Could you check a few things on this model? Use its own coordinates, in mm. Round coordinates to 2 decimals unless told otherwise and drop trailing zeros. Loops run counter-clockwise (first coordinate to the right, second up) from the corner with the lowest first, then second, coordinate; pieces in that order, holes last. Notation, with made-up numbers: M 45.25,41.25 L 50.25,41.25 A14 cw 50.25,54.25 Z; hole C -22.75,20 d8. An arc over 180 degrees is marked long. One line per item, written item: value. Start each with the question number.
Q1. Please list where these lines run through material, in increasing order: line 1 along X through (y, z) = (1.6, -32); line 2 along X through (y, z) = (1.35, -20.37); line 3 along X through (y, z) = (3, 19.63).
Q2. Imagine slicing it at D-D (z = 32). Please give me the cut outline in (x, y).
Q3. I'm going to push flat-ended pins straight in: pin 1 Ø2.5 at (x, z) = (58.87, -20.37) entering from +Y; pin 2 Ø2.5 at (x, y) = (-37.5, 1.5) entering from +Z; pin 3 Ø2.5 at (x, y) = (54.5, 3.5) entering from -Z; pin 4 Ø2.5 at (x, y) = (-70.5, 1.5) entering from -Z. Where does each tip first touch, or does it pass through?
Q4. Imagine slicing it at A-A (x = 1.5). Please give me the cut outline in (y, z), then the cut area to 3 significant figures.
Q5. Imagine slicing it at B-B (y = 3.3). Give the number of separate pieces and of enclosed holes in the cut face, then the cut area to 3 significant figures.
Q6. Imagine slicing it at C-C (x = 58.87). Please give me the cut outline in (y, z), then the cut area to 3 significant figures.
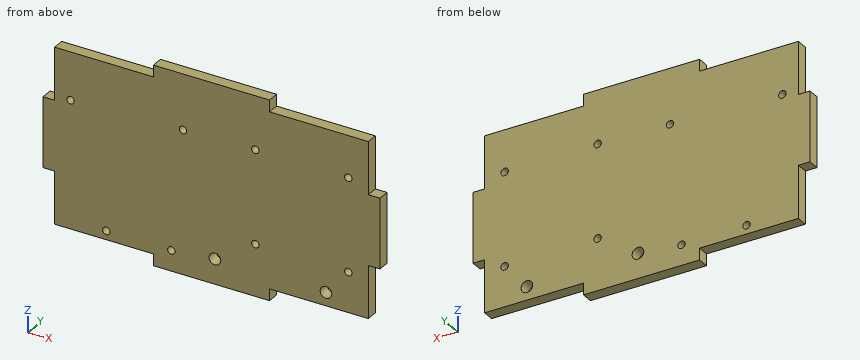
from build123d import *

# Parameters (mm, degrees)
SKETCH1_W           = 145
SKETCH1_H           = 85
BOSS_EXTRUDE1_DEPTH = 5
SKETCH2_W           = 47.5
SKETCH2_H           = 5
CUT_EXTRUDE1_DEPTH  = 5
SKETCH3_W           = 5
SKETCH3_H           = 22.5
CUT_EXTRUDE2_DEPTH  = 5
SKETCH4_R           = 1.6
CUT_EXTRUDE3_DEPTH  = 5
SKETCH5_R           = 1.6
CUT_EXTRUDE4_DEPTH  = 5
SKETCH6_R           = 2.5
CUT_EXTRUDE5_DEPTH  = 10


with BuildPart() as part:
    # Sketch1 → Boss-Extrude1 (new body)
    with BuildSketch(Plane(origin=(0, 0, 0), x_dir=(1, 0, 0), z_dir=(0, 1, 0))):
        Rectangle(SKETCH1_W, SKETCH1_H)
    extrude(amount=BOSS_EXTRUDE1_DEPTH)

    # Sketch2 → Cut-Extrude1 (cut)
    with BuildSketch(Plane(origin=(0, 5, 0), x_dir=(1, 0, 0), z_dir=(0, 1, 0))):
        with Locations((-48.75, 40)):
            Rectangle(SKETCH2_W, SKETCH2_H)
        with Locations((48.75, 40)):
            Rectangle(SKETCH2_W, SKETCH2_H)
        with Locations((48.75, -40)):
            Rectangle(SKETCH2_W, SKETCH2_H)
        with Locations((-48.75, -40)):
            Rectangle(SKETCH2_W, SKETCH2_H)
    extrude(amount=-CUT_EXTRUDE1_DEPTH, mode=Mode.SUBTRACT)

    # Sketch3 → Cut-Extrude2 (cut)
    with BuildSketch(Plane(origin=(0, 5, 0), x_dir=(1, 0, 0), z_dir=(0, 1, 0))):
        with Locations((-70, 26.25)):
            Rectangle(SKETCH3_W, SKETCH3_H)
        with Locations((-70, -26.25)):
            Rectangle(SKETCH3_W, SKETCH3_H)
        with Locations((70, -26.25)):
            Rectangle(SKETCH3_W, SKETCH3_H)
        with Locations((70, 26.25)):
            Rectangle(SKETCH3_W, SKETCH3_H)
    extrude(amount=-CUT_EXTRUDE2_DEPTH, mode=Mode.SUBTRACT)

    # Sketch4 → Cut-Extrude3 (cut)
    with BuildSketch(Plane(origin=(0, 5, 0), x_dir=(1, 0, 0), z_dir=(0, 1, 0))):
        with Locations(Location((-12.26, -18.77, 0), (0, 0, 270))):
            Circle(SKETCH4_R)
        with Locations(Location((-60.66, -17.06, 0), (0, 0, 270))):
            Circle(SKETCH4_R)
        with Locations(Location((-45.22, 33.75, 0), (0, 0, 270))):
            Circle(SKETCH4_R)
        with Locations(Location((-17.26, 33.75, 0), (0, 0, 270))):
            Circle(SKETCH4_R)
    extrude(amount=-CUT_EXTRUDE3_DEPTH, mode=Mode.SUBTRACT)

    # Sketch5 → Cut-Extrude4 (cut)
    with BuildSketch(Plane(origin=(0, 5, 0), x_dir=(1, 0, 0), z_dir=(0, 1, 0))):
        with Locations(Location((58.87, 20.37, 0), (0, 0, 270))):
            Circle(SKETCH5_R)
        with Locations(Location((18.87, 20.37, 0), (0, 0, 270))):
            Circle(SKETCH5_R)
        with Locations(Location((18.87, -19.63, 0), (0, 0, 270))):
            Circle(SKETCH5_R)
        with Locations(Location((58.87, -19.63, 0), (0, 0, 270))):
            Circle(SKETCH5_R)
    extrude(amount=-CUT_EXTRUDE4_DEPTH, mode=Mode.SUBTRACT)

    # Sketch6 → Cut-Extrude5 (cut)
    with BuildSketch(Plane(origin=(0, 5, 0), x_dir=(1, 0, 0), z_dir=(0, 1, 0))):
        with Locations(Location((49.29, 31.79, 0), (0, 0, 270))):
            Circle(SKETCH6_R)
        with Locations(Location((1.5, 31.79, 0), (0, 0, 270))):
            Circle(SKETCH6_R)
    extrude(amount=-CUT_EXTRUDE5_DEPTH, mode=Mode.SUBTRACT)


solid = part.part
Report:
1. line 1: x = -67.5 to -0.99, 3.99 to 46.8, 51.78 to 67.5
1. line 2: x = -67.5 to 17.27, 20.47 to 57.27, 60.47 to 67.5
1. line 3: x = -67.5 to -13.61, -10.91 to 17.27, 20.47 to 57.27, 60.47 to 67.5
2. outline: M -67.5,0 L 67.5,0 L 67.5,5 L -67.5,5 Z
3. pin 1: passes through
3. pin 2: stops at z = 37.5
3. pin 3: stops at z = -37.5
3. pin 4: stops at z = -15
4. outline: M 0,-42.5 L 5,-42.5 L 5,-34.29 L 0,-34.29 Z; M 0,-29.29 L 5,-29.29 L 5,42.5 L 0,42.5 Z
4. area: 400 mm²
5. separate pieces: 1
5. enclosed holes: 10
5. area: 10,800 mm²
6. outline: M 0,-37.5 L 5,-37.5 L 5,-21.97 L 0,-21.97 Z; M 0,-18.77 L 5,-18.77 L 5,18.03 L 0,18.03 Z; M 0,21.23 L 5,21.23 L 5,37.5 L 0,37.5 Z
6. area: 343 mm²
